Read the model definition and answer for the solid it produces. Units are mm, in the model's axes. A direction names the side the tool comes from. Coordinates: 2 decimals unless noted, no trailing zeros. Order: outer loops, then holes, each group sorted by start corner. A loop starts at its lowest first (then second) coordinate and runs counter-clockwise, first axis right, second up.
from build123d import *

# Parameters (mm, degrees)
BOSS_EXTRUDE1_DEPTH        = 39.878
F_10_32_TAPPED_HOLE1_D     = 4.0386
F_10_32_TAPPED_HOLE1_DEPTH = 39.878
F_6_32_TAPPED_HOLE1_D      = 2.7051
F_6_32_TAPPED_HOLE1_DEPTH  = 6.35
CUT_EXTRUDE1_REACH         = 12.319
SKETCH10_R                 = 3.96875


with BuildPart() as part:
    # Sketch1 → Boss-Extrude1 (new body)
    with BuildSketch(Plane(origin=(0, 0, 0), x_dir=(1, 0, 0), z_dir=(0, 1, 0))):
        Polygon((0, 0), (-3.96875, 0), (-3.96875, 9.525), (6.35, 9.525), (6.35, -10.31875), (0, -10.31875), align=None)
    extrude(amount=BOSS_EXTRUDE1_DEPTH)

    # #10-32 Tapped Hole1
    with Locations(Plane(origin=(0, 39.878, 0), x_dir=(1, 0, 0), z_dir=(0, 1, 0))):
        with Locations((1.11125, 4.7625)):
            Hole(F_10_32_TAPPED_HOLE1_D / 2, depth=F_10_32_TAPPED_HOLE1_DEPTH)

    # #6-32 Tapped Hole1
    with Locations(Plane.ZY):
        with Locations((5.159375, 13.97254)):
            Hole(F_6_32_TAPPED_HOLE1_D / 2, depth=F_6_32_TAPPED_HOLE1_DEPTH)

    # Sketch10 → Cut-Extrude1 (cut, up to next)
    with BuildSketch(Plane(origin=(6.35, 0, 0), x_dir=(0, 0, -1), z_dir=(1, 0, 0)), mode=Mode.PRIVATE) as cut_extrude1_sk1:
        with Locations((-5.159375, 24.47254)):
            Circle(SKETCH10_R)
    cut_extrude1_tool1 = extrude(cut_extrude1_sk1.sketch, amount=-CUT_EXTRUDE1_REACH, mode=Mode.PRIVATE) & part.part
    add(cut_extrude1_tool1.solids().sort_by_distance((6.35, 24.47254, 5.159375))[0], mode=Mode.SUBTRACT)


solid = part.part
Q1. The part is cut by section A-A, the plane y = 13.5. State how many separate pieces and enclosed holes the cut face has, then the cut area to 3 significant figures.
Q2. The part is cut by section B-B, the plane x = 2.5. Determine the outline of the cut face in (y, z) (1 decimal), then the cut area to 3 significant figures.
Q3. This flat-tipped pin is pushed along its axis until it touches: P1, Ø2, axis at y = 35.5, z = 7.5, coming from the -X side. Where does it stop, or does it pass through?
Q4. The part is cut by section C-C, the plane z = 8. Determine the outline of the cut face in (x, y), then the cut area to 3 significant figures.
Q5. Determine the mould class of faces 1 (the flat face through (2, 0, 0)), 2 (the cylindrical face through (3.22, 15.11, 4.43)), 3 (the flat face through (3, 20, 10.319)) for opening direction Y: +Y half, -Y half, draft (parallel to the pull), parting line (faces both ways), or undercut.
Q6. Straight lines are drawn through the part: L1, parallel to Z at x = 4.75, y = 24.5 (3 decimals); L2, parallel to Z at x = 5, y = 14 (3 decimals); L3, parallel to Z at x = -1.5, y = 27 (3 decimals). For each, find the intervals that lie inside material, in ascending order.
Q7. Which of the six approach directions +Z, -Z, +X, -X, +Y, -Y give full straight-line access (tool end or side, diameter ignored) to faces 4 (the flat face through (-2, 20, 0)), 5 (the flat face through (6.35, 20, 0))?
Computed values:
1. separate pieces: 2
1. enclosed holes: 1
1. area: 135 mm2
2. outline: (0, -9.5) - (39.9, -9.5) - (39.9, -6.2) - (0, -6.2) - close; (0, -3.3) - (39.9, -3.3) - (39.9, 10.3) - (0, 10.3) - close; hole circle Ø2.7 at (14, 5.2); hole circle Ø7.9 at (24.5, 5.2)
2. area: 619 mm2
3. P1: stops at x = 0
4. outline: (0, 0) - (6.35, 0) - (6.35, 21.7) - (0, 21.7) - close; (0, 27.24) - (6.35, 27.24) - (6.35, 39.88) - (0, 39.88) - close
4. area: 218 mm2
5. face 1: -Y half
5. face 2: undercut
5. face 3: draft
6. L1: z = -9.525 to 1.191, 9.128 to 10.319
6. L2: z = -9.525 to 3.807, 6.512 to 10.319
6. L3: z = -9.525 to 0
7. face 4: +Z, -X, +Y, -Y
7. face 5: +Z, -Z, +X, +Y, -Y
